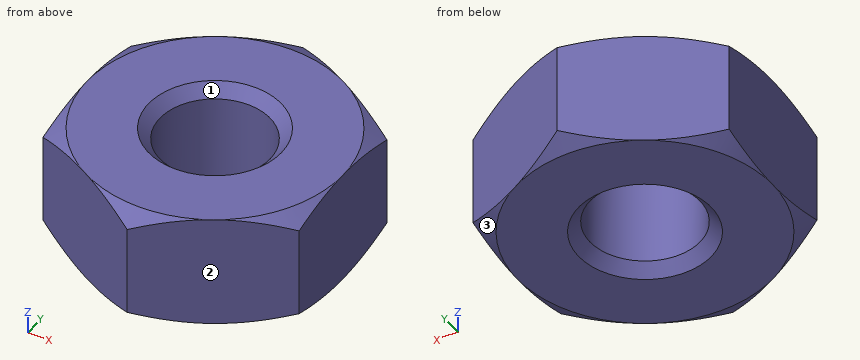
from build123d import *

# Parameters (mm, degrees)
F0_R     = 12.423166
F1_DEPTH = 25.4
F4_SIZE  = 2.54
F5_SIZE  = 2.54


with BuildPart() as f1:
    # F0 (on Top) → F1 (new body)
    with BuildSketch(Plane.XY):
        Polygon((-28.755525, 16.60201), (-28.755525, -16.60201), (0, -33.20402), (28.755525, -16.60201), (28.755525, 16.60201), (0, 33.20402), align=None)
        Circle(F0_R, mode=Mode.SUBTRACT)
    extrude(amount=F1_DEPTH)

    # F2 (on Front) → F3 (revolve, cut)
    with BuildSketch(Plane.XZ):
        Polygon((-47.010668, 14.860389), (-28.755525, 25.4), (-47.010668, 25.4), align=None)
        Polygon((-47.010668, 0), (-28.755525, 0), (-47.010668, 10.539611), align=None)
    revolve(axis=Axis((0, 0, 12.7), (0, 0, 1)), mode=Mode.SUBTRACT)

    # F4
    f4_edges = [f1.edges().sort_by_distance(p)[0] for p in [
        (-12.423166, 0, 25.4),
    ]]
    chamfer(f4_edges, length=F4_SIZE)

    # F5
    f5_edges = [f1.edges().sort_by_distance(p)[0] for p in [
        (-12.423166, 0, 0),
    ]]
    chamfer(f5_edges, length=F5_SIZE)


solid = f1.part
CAD build for the part. Positions are in the model's coordinates, mm. Face numbers are marked on the shaded views. Give positions to 0.01 mm unless a question says otherwise; leave off trailing zeros. Loops run counter-clockwise (first coordinate to the right, second up) from the corner with the lowest first, then second, coordinate; pieces in that order, holes last. Notation, with made-up numbers: M 43.5,-30.75 L 101.5,-30.75 A22 cw 101.5,-9.75 Z; hole C 31.25,47.5 d7. An arc over 180 degrees is marked long. One line per question, with ' | ' between items. Start each with the question number.
1. Two-plate mould, pull along Y, no slides. Class the marked faces 1, 2 and 3: pulls with the +Y half, pulls with the -Y half, needs draft (parallel to the pull), parting line crosses it, or undercut.
2. Saw through at A-A on z = 4. Give the cut face in (x, y), plus the area to 3 significant figures.
3. Flat gauge pins, fed straight in: pin 1 (1 mm diameter, centred on x = -7, z = 16.5, fed in from +Y); pin 2 (2 mm diameter, centred on x = -9.5, z = 13, fed in from +Y); pin 3 (12 mm diameter, centred on x = 0.5, y = -12, fed in from -Z); pin 4 (15 mm diameter, centred on x = 0, y = 0, fed in from +Z). Where does each tip first touch, or does it go through?
4. Probe L1, parallel to Y at x = 0, z = 9.75; L2, parallel to Y at x = -5.5, z = 9.25; L3, parallel to Y at x = -12.5, z = 12.5. List the from-to ranges inside material, lowest first. Write a range as from..to.
Result sheet:
1) face 1: undercut | face 2: pulls with the -Y half | face 3: pulls with the +Y half
2) outline: M -28.76,-16.6 L 0,-33.2 L 28.76,-16.6 L 28.76,16.6 L 0,33.2 L -28.76,16.6 Z; hole C 0,0 d24.85 | area: 2,380 mm^2
3) pin 1: stops at y = 29.45 | pin 2: stops at y = 28.3 | pin 3: stops at z = 0 | pin 4: passes through
4) L1: y = -33.2..-12.42, 12.42..33.2 | L2: y = -30.03..-11.14, 11.14..30.03 | L3: y = -25.99..25.99
